CAD build for the part. Positions are in the model's coordinates, mm. Face numbers are marked on the shaded views. Give positions to 0.01 mm unless a question says otherwise; leave off trailing zeros. Write each loop counter-clockwise with the first axis right and the second up, starting at its lowest first coordinate (ties: lowest second). Pieces come first, ordered by that corner, then holes. Notation, with made-up numbers: (55.25, 13) - (109.25, 13) arc R15 cw to (109.25, 29) - close; hole circle Ø1 at (36.25, 44). An arc over 180 degrees is marked (long way). Put each result on its own line as item: value. Start each with the question number.
1. Mould opens along X. For the marked faces 1, 2, 3 and 4 say: +X half, -X half, draft (parallel to the pull), parting line (faces both ways), or undercut.
2. Wall check: line 1 (Y direction, x = 0, z = -7.5); line 2 (Y direction, x = 0, z = -14); line 3 (Y direction, x = -1.25, z = -10). Give the ranges that are in metal, low to high.
3. Cut at A-A on y = 12.7. List the corners of the cut face in (x, z), and give its area (3 significant figures).
4. Cut at D-D on y = 15.5. List the corners of the cut face in (x, z), and give its area (3 significant figures).
5. Cut at B-B on z = -12.7. Give the number of separate pieces and of enclosed holes in the cut face, and give its area (3 significant figures).
6. Drop flat-ended pins along their axis: pin 1 (4 mm diameter, centred on y = 13, z = -10, fed in from -X); pin 2 (5 mm diameter, centred on x = -3.5, z = -8.5, fed in from -Y); pin 3 (1 mm diameter, centred on x = 2.5, z = -4.5, fed in from -Y). Give the stop position or say it passes through.
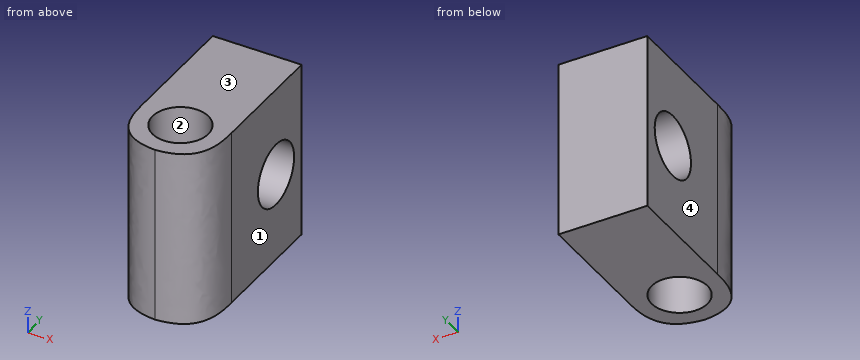
from build123d import *

# Parameters (mm, degrees)
SKETCH1_W           = 12.7
SKETCH1_H           = 12.7
SKETCH1_R           = 3.9878
BOSS_EXTRUDE1_DEPTH = 25.4
SKETCH2_R           = 4.49961
CUT_EXTRUDE1_DEPTH  = 12.7
FILLET1_SIZE        = 7.9756


with BuildPart() as part:
    # Sketch1 → Boss-Extrude1 (new body)
    # profile 1 of 2: a face of its own
    with BuildSketch(Plane.XY):
        with Locations((0, 12.7)):
            Rectangle(SKETCH1_W, SKETCH1_H)
    # profile 2 of 2: a face of its own
    with BuildSketch(Plane.XY):
        Rectangle(SKETCH1_W, SKETCH1_H)
        Circle(SKETCH1_R, mode=Mode.SUBTRACT)
    extrude(amount=-BOSS_EXTRUDE1_DEPTH)

    # Sketch2 → Cut-Extrude1 (cut)
    with BuildSketch(Plane.ZY.offset(6.35)):
        with Locations((-12.7, 12.7)):
            Circle(SKETCH2_R)
    extrude(amount=-CUT_EXTRUDE1_DEPTH, mode=Mode.SUBTRACT)

    # Fillet1
    # a fillet whose section is not a circle: 7.9756 mm, written as the material it takes off along each edge
    with BuildSketch(Plane(origin=(-6.35, -6.35, 19.939), x_dir=(1, 0, 0), z_dir=(0, 0, -1)), Plane(origin=(6.35, -6.35, 19.939), x_dir=(0, 1, 0), z_dir=(0, 0, -1))) as fillet1_piece_1:
        with BuildLine():
            add(Edge.make_bspline([(FILLET1_SIZE, 0), (FILLET1_SIZE * 0.831801948466, 0), (FILLET1_SIZE * 0.663603896932, 0), (FILLET1_SIZE * 0.292893218813, -FILLET1_SIZE * 0.0716919198361), (FILLET1_SIZE * 0.0716919198361, -FILLET1_SIZE * 0.292893218813), (0, -FILLET1_SIZE * 0.663603896932), (0, -FILLET1_SIZE * 0.831801948466), (0, -FILLET1_SIZE)], knots=[0, 0, 0, 0, 0, 0, 0.5, 0.5, 1, 1, 1, 1, 1, 1], degree=5))
            Line((0, -FILLET1_SIZE), (0, 0))
            Line((0, 0), (FILLET1_SIZE, 0))
        make_face()
    extrude(amount=65.278, mode=Mode.SUBTRACT)


solid = part.part
Report:
1. face 1: +X half
1. face 2: undercut
1. face 3: draft
1. face 4: -X half
2. line 1: y = -6.31 to -3.99, 3.99 to 19.05
2. line 2: y = -6.31 to -3.99, 3.99 to 8.39, 17.01 to 19.05
2. line 3: y = -6.17 to -3.79, 3.79 to 9.1, 16.3 to 19.05
3. outline: (-6.35, -25.4) - (6.35, -25.4) - (6.35, -17.2) - (-6.35, -17.2) - close; (-6.35, -8.2) - (6.35, -8.2) - (6.35, 0) - (-6.35, 0) - close
3. area: 208 mm²
4. outline: (-6.35, -25.4) - (6.35, -25.4) - (6.35, -16.22) - (-6.35, -16.22) - close; (-6.35, -9.18) - (6.35, -9.18) - (6.35, 0) - (-6.35, 0) - close
4. area: 233 mm²
5. separate pieces: 2
5. enclosed holes: 1
5. area: 142 mm²
6. pin 1: stops at x = -6.35
6. pin 2: stops at y = -6.21
6. pin 3: stops at y = -6.01
